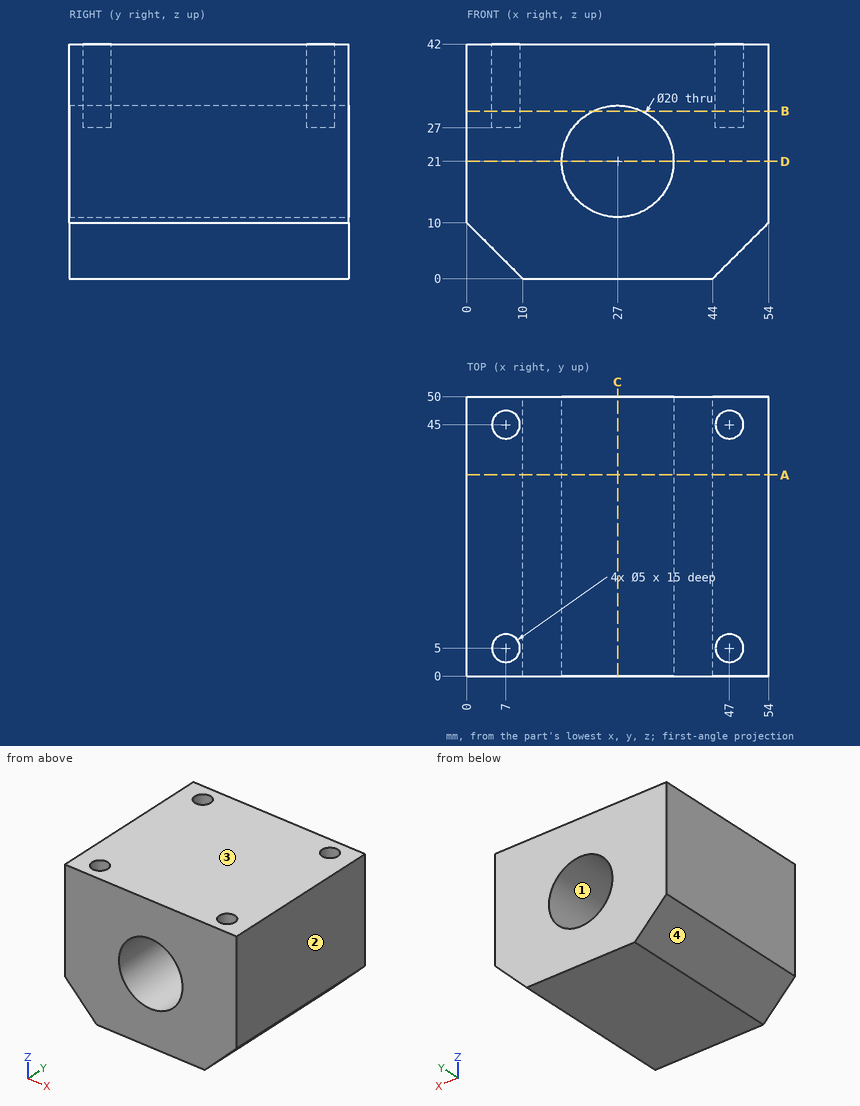
Check sheet for the drawn part. Datum: minimum x, y, z corner. Units: mm. Round coordinates to 2 decimals unless told otherwise and drop trailing zeros. Loops run counter-clockwise (first coordinate to the right, second up) from the corner with the lowest first, then second, coordinate; pieces in that order, holes last.
Item 1: Gauge pin test, flat ends, axial feed: pin 1 (3 mm diameter, centred on x = 7, y = 5, fed in from +Z); pin 2 (12 mm diameter, centred on x = 27, z = 21, fed in from -Y); pin 3 (4 mm diameter, centred on x = 47, y = 45, fed in from -Z). Record the tip position at first contact, or that the pin passes through.
Item 2: Mould release check, pull along Z, two halves, no side actions. Record for the marked faces 1, 2, 3 and 4: pulls with the +Z half, pulls with the -Z half, needs draft (parallel to the pull), parting line crosses it, or undercut.
Item 3: Cross-section at B-B on z = 30. Record the boundary of the cut face in (x, y).
Item 4: Cross-section at C-C on x = 27. Record the boundary of the cut face in (y, z), then the cut area to 3 significant figures.
Item 5: Cross-section at D-D on z = 21. Record the boundary of the cut face in (x, y).
Item 6: Thickness scan on line 1 (Y direction, x = 47, z = 34); line 2 (Y direction, x = 45, z = 31.5); line 3 (Z direction, x = 46.5, y = 2). Record the ranges inside material, lowest first.
Item 7: Cross-section at A-A on y = 36. Record the boundary of the cut face in (x, z), then the cut area to 3 significant figures.
Answer sheet:
1. pin 1: stops at z = 27
1. pin 2: passes through
1. pin 3: stops at z = 1
2. face 1: undercut
2. face 2: needs draft
2. face 3: pulls with the +Z half
2. face 4: pulls with the -Z half
3. outline: (0, 0) - (22.64, 0) - (22.64, 50) - (0, 50) - close; (31.36, 0) - (54, 0) - (54, 50) - (31.36, 50) - close; hole circle Ø5 at (7, 5); hole circle Ø5 at (7, 45); hole circle Ø5 at (47, 5); hole circle Ø5 at (47, 45)
4. outline: (0, 0) - (50, 0) - (50, 11) - (0, 11) - close; (0, 31) - (50, 31) - (50, 42) - (0, 42) - close
4. area: 1,100 mm2
5. outline: (0, 0) - (17, 0) - (17, 50) - (0, 50) - close; (37, 0) - (54, 0) - (54, 50) - (37, 50) - close
6. line 1: y = 0 to 2.5, 7.5 to 42.5, 47.5 to 50
6. line 2: y = 0 to 3.5, 6.5 to 43.5, 46.5 to 50
6. line 3: z = 2.5 to 42
7. outline: (0, 10) - (10, 0) - (44, 0) - (54, 10) - (54, 42) - (0, 42) - close; hole circle Ø20 at (27, 21)
7. area: 1,850 mm2
